Work out the finished part from the listing and answer in its coordinate system (mm). Face numbers are marked on the shaded views. A direction names the side the tool comes from. Coordinates: 2 decimals unless noted, no trailing zeros. Loops run counter-clockwise (first coordinate to the right, second up) from the corner with the lowest first, then second, coordinate; pieces in that order, holes last. Notation, with made-up numbers: (-29.75, 74) -> (25.25, 74) arc R29 ccw to (25.25, 98) -> close; hole circle Ø11 at (56, 63.5). An arc over 180 degrees is marked (long way). One line per question, with ' | ' between items.
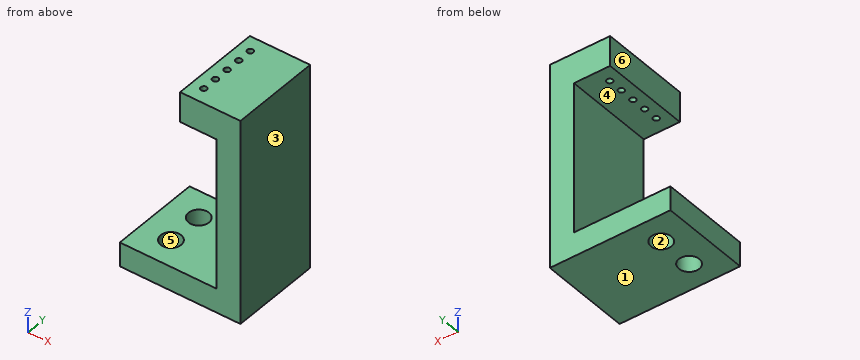
```python
from build123d import *

# Parameters (mm, degrees)
F0_W     = 16
F0_H     = 15
F0_R     = 1.7
F0_W_2   = 4
F1_DEPTH = 4
F2_DEPTH = 25
F3_W     = 10
F3_H     = 15
F3_R     = 0.5
F4_DEPTH = 5


with BuildPart() as f1:
    # F0 (on Top) → F1 (new body)
    with BuildSketch(Plane.XY):
        with Locations((-12, 0)):
            Rectangle(F0_W, F0_H)
        with Locations((-15, -3)):
            Circle(F0_R, mode=Mode.SUBTRACT)
        with Locations((-15, 3)):
            Circle(F0_R, mode=Mode.SUBTRACT)
        with Locations((-2, 0)):
            Rectangle(F0_W_2, F0_H)
    extrude(amount=-F1_DEPTH)

    # F0 (on Top) → F2 (join)
    with BuildSketch(Plane.XY):
        with Locations((-2, 0)):
            Rectangle(F0_W_2, F0_H)
    extrude(amount=F2_DEPTH)

    # F3 (on face) → F4 (join)
    with BuildSketch(Plane.XY.offset(25)):
        with Locations((-5, 0)):
            Rectangle(F3_W, F3_H)
        with Locations((-8, -5)):
            Circle(F3_R, mode=Mode.SUBTRACT)
        with Locations((-8, -2.5)):
            Circle(F3_R, mode=Mode.SUBTRACT)
        with Locations((-8, 0)):
            Circle(F3_R, mode=Mode.SUBTRACT)
        with Locations((-8, 2.5)):
            Circle(F3_R, mode=Mode.SUBTRACT)
        with Locations((-8, 5)):
            Circle(F3_R, mode=Mode.SUBTRACT)
    extrude(amount=F4_DEPTH)


solid = f1.part
```
1) For the marked faces 4, 5 and 6, determine the directions among +Z, -Z, +X, -X, +Y, -Y from which every point of the face is accessible in a straight line to the end or side of a thin tool.
Check values:
face 4: -X, +Y, -Y | face 5: +Z, -Z | face 6: +Z, -X, +Y, -Y
2) Find section B-B (y = 0). Write down the section's boundary in (x, z), plus the area to 3 significant figures.
Check values:
outline: (-20, -4) -> (0, -4) -> (0, 30) -> (-7.5, 30) -> (-7.5, 25) -> (-4, 25) -> (-4, 0) -> (-20, 0) -> close; (-10, 25) -> (-8.5, 25) -> (-8.5, 30) -> (-10, 30) -> close | area: 225 mm^2
3) Flat-ended cylindrical pins translate along their axes: pin 1 (2.5 mm diameter, centred on y = -0.5, z = 27.5, fed in from -X); pin 2 (4.5 mm diameter, centred on x = -15, y = -3.5, fed in from +Z); pin 3 (6 mm diameter, centred on y = -0.5, z = 16.5, fed in from -X). Find the tip coordinate at first contact, or state that the pin passes through.
Check values:
pin 1: stops at x = -10 | pin 2: stops at z = 0 | pin 3: stops at x = -4
4) Find section A-A (x = -6.25). Write down the section's boundary in (y, z).
Check values:
outline: (-7.5, -4) -> (7.5, -4) -> (7.5, 0) -> (-7.5, 0) -> close; (-7.5, 25) -> (7.5, 25) -> (7.5, 30) -> (-7.5, 30) -> close
5) The mould has two halves that part along X. Classify the marked faces 1, 2 and 3: released by +X, released by -X, zero draft, split by the parting line, or undercut.
Check values:
face 1: zero draft | face 2: undercut | face 3: released by +X
6) Find section C-C (x = -15). Write down the section's boundary in (y, z), plus the area to 3 significant figures.
Check values:
outline: (-7.5, -4) -> (-4.7, -4) -> (-4.7, 0) -> (-7.5, 0) -> close; (-1.3, -4) -> (1.3, -4) -> (1.3, 0) -> (-1.3, 0) -> close; (4.7, -4) -> (7.5, -4) -> (7.5, 0) -> (4.7, 0) -> close | area: 32.8 mm^2
7) Find the intervals of material crossed by line 1 along Y through (x, z) = (-15, -1.25); line 2 along Z through (x, y) = (-5, -3); line 3 along X through (y, z) = (-4.5, 22.5), in increasing order.
Check values:
line 1: y = -7.5 to -4.7, -1.3 to 1.3, 4.7 to 7.5 | line 2: z = -4 to 0, 25 to 30 | line 3: x = -4 to 0
8) Find section D-D (y = -2.5). Write down the section's boundary in (x, z).
Check values:
outline: (-20, -4) -> (-16.62, -4) -> (-16.62, 0) -> (-20, 0) -> close; (-13.38, -4) -> (0, -4) -> (0, 30) -> (-7.5, 30) -> (-7.5, 25) -> (-4, 25) -> (-4, 0) -> (-13.38, 0) -> close; (-10, 25) -> (-8.5, 25) -> (-8.5, 30) -> (-10, 30) -> close
